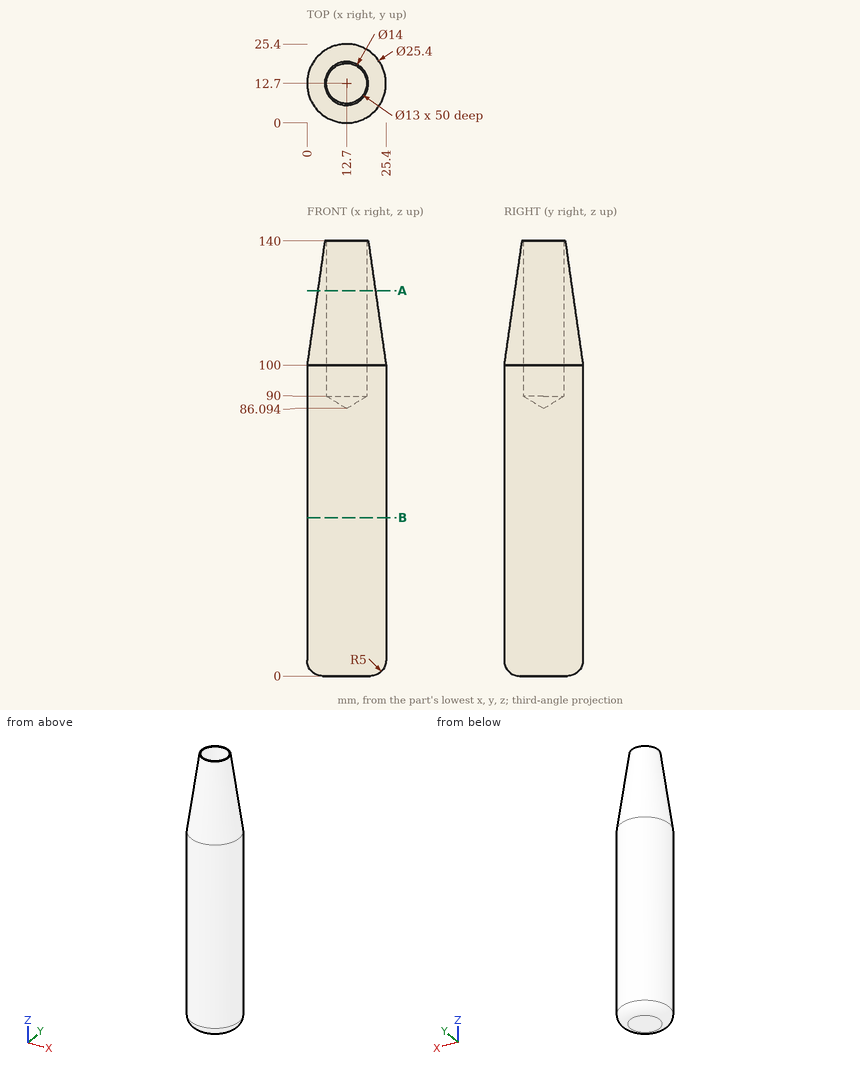
For this review, use the dimensioned drawing (mm, ordinates from the lowest corner) and the shaded views. Coordinates: 2 decimals unless noted, no trailing zeros. Write each loop counter-clockwise with the first axis right and the second up, starting at its lowest first coordinate (ties: lowest second). Pieces come first, ordered by that corner, then holes. Notation, with made-up numbers: (82, 6.5) - (101, 6.5) arc R35 ccw to (101, 39.5) - close; hole circle Ø6 at (12, -24.5). An arc over 180 degrees is marked (long way). Answer as a JSON object with one key per item and string values. Group by question number.
1. Add section B-B (z = 51). Give the boundary of the cut face in (x, y), plus the area to 3 significant figures.
2. To check wall thickness, follow probe 1 along Y at (x, z) = (12.7, 116); probe 2 along X at (y, z) = (12.7, 121); probe 3 along Y at (x, z) = (12.7, 112.5). State the ranges of each line that lie inside material, in increasing order.
3. Clearance check with flat-ended pins moving along their axes: pin 1 Ø2 at (x, y) = (13.5, 16.5) entering from +Z; pin 2 Ø5 at (y, z) = (12, 107.5) entering from -X; pin 3 Ø12 at (x, y) = (9, 10.5) entering from +Z; pin 4 Ø8 at (x, y) = (12.7, 12.7) entering from +Z. State where each tip first meets the part, or that it passes through.
4. Add section A-A (z = 124). Give the boundary of the cut face in (x, y).
Findings:
{
 "1": {"outline": "circle Ø25.4 at (12.7, 12.7)", "area": "507 mm²"},
 "2": {"probe 1": "2.28 to 6.2, 19.2 to 23.12", "probe 2": "2.99 to 6.2, 19.2 to 22.41", "probe 3": "1.78 to 6.2, 19.2 to 23.62"},
 "3": {"pin 1": "z = 89.03", "pin 2": "x = 0.72", "pin 3": "z = 140", "pin 4": "z = 88.5"},
 "4": {"outline": "circle Ø18.56 at (12.7, 12.7); hole circle Ø13 at (12.7, 12.7)"}
}
